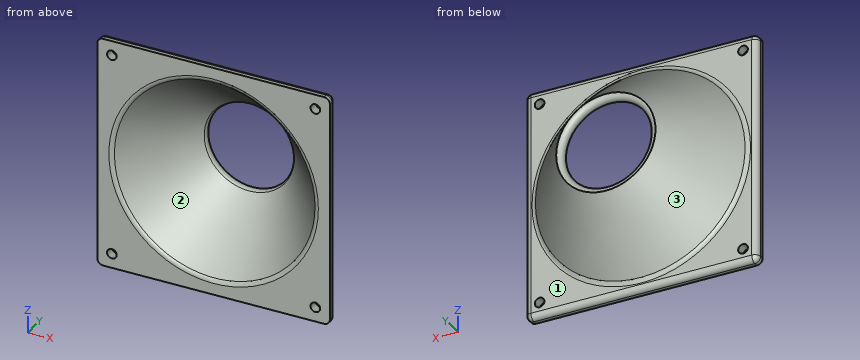
from build123d import *

# Parameters (mm, degrees)
SKETCH1_W           = 120
SKETCH1_H           = 120
SKETCH1_R           = 2.5
BOSS_EXTRUDE1_DEPTH = 5
SKETCH2_R           = 55
BOSS_EXTRUDE2_DEPTH = 35
BOSS_EXTRUDE2_TAPER = 40
FILLET1_R           = 3
FILLET2_R           = 3
FILLET3_R           = 3


# Read off the part's stored shape, not the designer's step: Shell1
with BuildPart() as part:
    # Sketch1 → Boss-Extrude1 (new body)
    with BuildSketch(Plane(origin=(0, 0, 0), x_dir=(1, 0, 0), z_dir=(0, 1, 0))):
        Rectangle(SKETCH1_W, SKETCH1_H)
        with Locations(Location((-52.5, 52.5, 0), (0, 0, 270))):
            Circle(SKETCH1_R, mode=Mode.SUBTRACT)
        with Locations(Location((52.5, 52.5, 0), (0, 0, 270))):
            Circle(SKETCH1_R, mode=Mode.SUBTRACT)
        with Locations(Location((52.5, -52.5, 0), (0, 0, 270))):
            Circle(SKETCH1_R, mode=Mode.SUBTRACT)
        with Locations(Location((-52.5, -52.5, 0), (0, 0, 270))):
            Circle(SKETCH1_R, mode=Mode.SUBTRACT)
    extrude(amount=BOSS_EXTRUDE1_DEPTH)

    # Sketch2 → Boss-Extrude2 (add)
    with BuildSketch(Plane(origin=(0, 5, 0), x_dir=(1, 0, 0), z_dir=(0, 1, 0))):
        Circle(SKETCH2_R)
    extrude(amount=BOSS_EXTRUDE2_DEPTH, taper=BOSS_EXTRUDE2_TAPER)

    # Shell1 outline → Shell1 (revolve, cut)
    with BuildSketch(Plane.XY):
        Polygon((0, 0), (52.668461709, 0), (19.104476462, 40), (0, 40), align=None)
    revolve(axis=Axis((0, 0, 0), (0, 1, 0)), mode=Mode.SUBTRACT)

    # Fillet1
    fillet1_edges = [part.edges().sort_by_distance(p)[0] for p in [
        (-55, 5, 0),
        (-19.104476462, 40, 0),
    ]]
    fillet(fillet1_edges, radius=FILLET1_R)

    # Fillet2
    fillet2_edges = [part.edges().sort_by_distance(p)[0] for p in [
        (-52.668461709, 0, 0),
    ]]
    fillet(fillet2_edges, radius=FILLET2_R)

    # Fillet3
    fillet3_edges = [part.edges().sort_by_distance(p)[0] for p in [
        (-60, 5, 0),
        (0, 5, 60),
        (60, 5, 0),
        (60, 2.5, 60),
        (-60, 2.5, 60),
        (-60, 2.5, -60),
        (60, 2.5, -60),
        (0, 5, -60),
    ]]
    fillet(fillet3_edges, radius=FILLET3_R)


solid = part.part
Design review of the part built by this model. Coordinates are the model's own, in mm. Face numbers are marked on the shaded views. Coordinates: 2 decimals unless noted, no trailing zeros. Loops run counter-clockwise (first coordinate to the right, second up) from the corner with the lowest first, then second, coordinate; pieces in that order, holes last. Notation, with made-up numbers: M 86.25,76.5 L 91.25,76.5 A24 cw 91.25,95.5 Z; hole C -38.5,-25.5 d8. An arc over 180 degrees is marked long. Answer as CSV lines item,"result".
Item 1: Add section A-A on x = 0. State the section outline as (y, z) points, plus the area to 3 significant figures.
Answer list:
outline,"M 0,-60 L 2,-60 A3 ccw 5,-57 L 5,-56.4 A3 cw 6.07,-54.1 L 40,-25.63 L 40,-25.54 A3 ccw 35.07,-23.24 L 1.07,-51.77 A3 ccw 0,-54.07 Z; M 0,54.07 A3 ccw 1.07,51.77 L 35.07,23.24 A3 ccw 40,25.54 L 40,25.63 L 6.07,54.1 A3 cw 5,56.4 L 5,57 A3 ccw 2,60 L 0,60 Z"
area,"529 mm²"
Item 2: Add section C-C on y = 11. State the section outline as (x, z) points, plus the area to 3 significant figures.
Answer list:
outline,"C 0,0 d99.93; hole C 0,0 d86.88"
area,"1,920 mm²"
Item 3: Add section B-B on y = 3.5. State the section outline as (x, z) points.
Answer list:
outline,"M -59.6,-57 A2.6 ccw -57,-59.6 L 57,-59.6 A2.6 ccw 59.6,-57 L 59.6,57 A2.6 ccw 57,59.6 L -57,59.6 A2.6 ccw -59.6,57 Z; hole C -52.5,-52.5 d5; hole C -52.5,52.5 d5; hole C 0,0 d99.46; hole C 52.5,-52.5 d5; hole C 52.5,52.5 d5"
Item 4: For P1, Ø8, axis at x = -29, y = 7, coming from the +Z side; P2, Ø5, axis at y = 20.5, z = 3, coming from the -X side; P3, Ø4, axis at x = -52.5, z = 52.5, coming from the +Y side (3 decimals); P4, Ø3, axis at x = -39, z = 11.5, coming from the -Y side, all flat-tipped, find the tip position at first contact; note any pin that passes through.
Answer list:
P1,"z = 59.83"
P2,"x = -44"
P3,"through"
P4,"y = 12.52"
Item 5: The part is to be moulded in two halves that separate along Z. For the marked faces 1, 2 and 3, say which applies: pulls with the +Z half, pulls with the -Z half, needs draft (parallel to the pull), parting line crosses it, or undercut.
Answer list:
face 1,"needs draft"
face 2,"undercut"
face 3,"parting line crosses it"
Item 6: Add section D-D on y = 24. State the section outline as (x, z) points, plus the area to 3 significant figures.
Answer list:
outline,"C 0,0 d78.11; hole C 0,0 d65.06"
area,"1,470 mm²"
Item 7: For probe 1 along X at (y, z) = (1.3, -52.5); probe 2 along Z at (x, y) = (52, 3); probe 3 along X at (y, z) = (3.8, -52.5), list the stretches that pass through material, from the lowest coordinate up.
Answer list:
probe 1,"-60 to -55, -50 to 50, 55 to 60"
probe 2,"-59.83 to -54.95, -50.05 to 50.05, 54.95 to 59.83"
probe 3,"-59.4 to -55, -50 to 50, 55 to 59.4"
